Can you work these out from the drawing? Everything is in mm from the part's minimum corner. Round coordinates to 2 decimals unless told otherwise and drop trailing zeros. Answer in a Markdown table with one row per item. Add a question column.
(1) I'm going to push a flat-ended pin straight in: pin 1 (5 mm diameter, centred on x = 42, y = 80, fed in from -Z). Where does the tip first touch, or does it pass through?
(2) If we mould it in two halves opening along X, with no side actions, what happens to the marked faces 1, 2 and 3? For each: released by +X, released by -X, zero draft, split by the parting line, or undercut.
(3) If I drill on probe 1 along Y at (x, z) = (62.5, 99.5) (1 decimal); probe 2 along Y at (x, z) = (41, 54.5) (1 decimal); probe 3 along X at (y, z) = (53.5, 78) (1 decimal), over which ranges is the centre line in solid material (lowest first)?
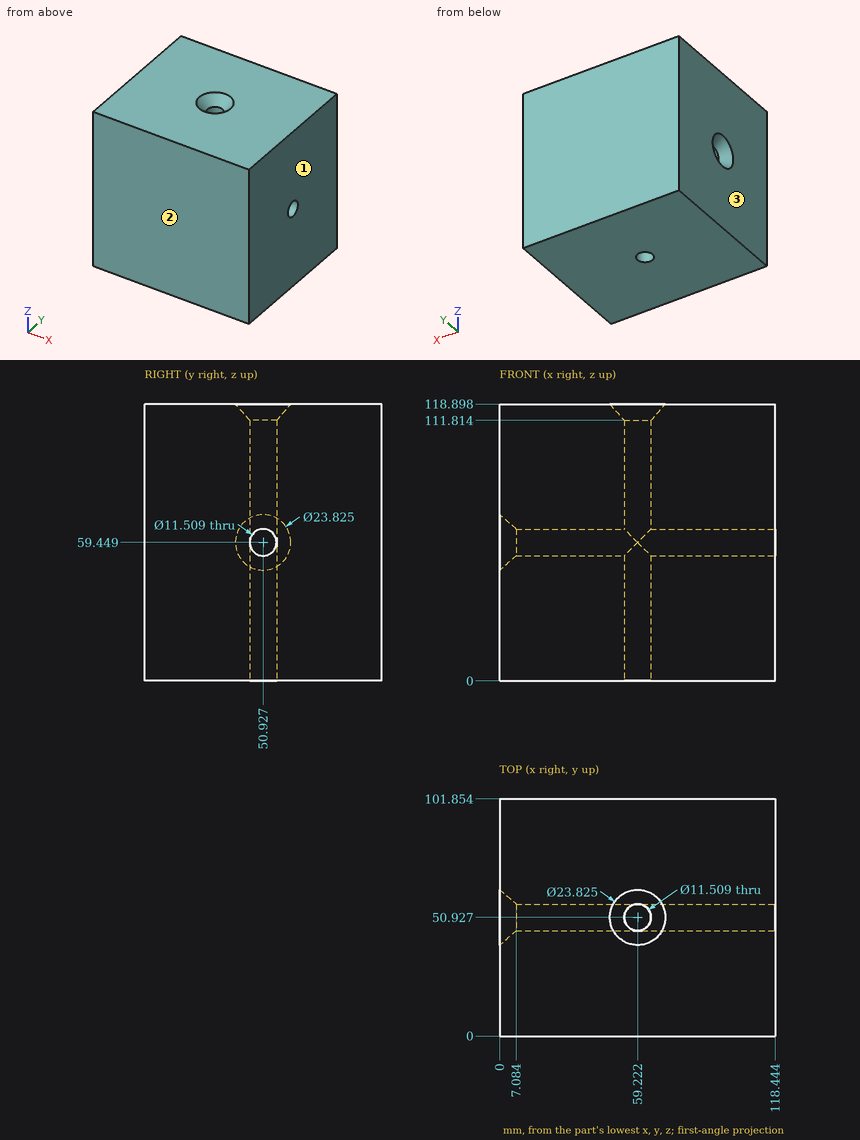
Calculated:
| question | item | result |
|---|---|---|
| 1 | pin 1 | z = 0 |
| 2 | face 1 | released by +X |
| 2 | face 2 | zero draft |
| 2 | face 3 | released by -X |
| 3 | probe 1 | 0 to 46.2, 55.7 to 101.9 |
| 3 | probe 2 | 0 to 48, 53.9 to 101.9 |
| 3 | probe 3 | 0 to 54.1, 64.4 to 118.4 |
